The model under review builds one solid part; all positions refer to its coordinate system, in mm. A direction names the side the tool comes from. Coordinates: 2 decimals unless noted, no trailing zeros. Write each loop counter-clockwise with the first axis right and the second up, starting at its lowest first coordinate (ties: lowest second). Pieces come first, ordered by that corner, then holes. Notation, with made-up numbers: (-9.75, 7) -> (9.25, 7) arc R21 ccw to (9.25, 36) -> close; hole circle Ø6 at (67, 69). An arc over 180 degrees is marked (long way). Write each question's results on one line, items separated by ' | '.
```python
from build123d import *

# Parameters (mm, degrees)
F0_W     = 80
F0_H     = 180
F1_DEPTH = 15
F2_W     = 50
F2_H     = 2
F3_DEPTH = 180
F4_ANGLE = 90
F5_ANGLE = 90
F6_DEPTH = 25
F9_DEPTH = 80.001


with BuildPart() as f1:
    # F0 (on Top) → F1 (new body)
    with BuildSketch(Plane.XY):
        Rectangle(F0_W, F0_H)
    extrude(amount=F1_DEPTH)

    # F2 (on face) → F3 (intersect, through all)
    with BuildSketch(Plane.XZ.offset(90)):
        with BuildLine():
            Line((-38, 15), (-40, 15))
            ThreePointArc((-40, 15), (-35.6066017178, 4.3933982822), (-25, 0))
            Line((-25, 0), (-25, 2))
            ThreePointArc((-25, 2), (-34.1923881554, 5.8076118446), (-38, 15))
        make_face()
        with Locations((0, 1)):
            Rectangle(F2_W, F2_H)
        with BuildLine():
            Line((25, 2), (25, 0))
            ThreePointArc((25, 0), (35.6066017178, 4.3933982822), (40, 15))
            Line((40, 15), (38, 15))
            ThreePointArc((38, 15), (34.1923881554, 5.8076118446), (25, 2))
        make_face()
    extrude(amount=-F3_DEPTH, mode=Mode.INTERSECT)

    # F2 (on face) → F4 (revolve)
    with BuildSketch(Plane.XZ.offset(90)):
        with BuildLine():
            Line((25, 2), (25, 0))
            ThreePointArc((25, 0), (35.6066017178, 4.3933982822), (40, 15))
            Line((40, 15), (38, 15))
            ThreePointArc((38, 15), (34.1923881554, 5.8076118446), (25, 2))
        make_face()
    revolve(axis=Axis((12.5, -90, 8.5), (0, 0, -1)), revolution_arc=F4_ANGLE)

    # F2 (on face) → F5 (revolve)
    with BuildSketch(Plane.XZ.offset(90)):
        with BuildLine():
            Line((-38, 15), (-40, 15))
            ThreePointArc((-40, 15), (-35.6066017178, 4.3933982822), (-25, 0))
            Line((-25, 0), (-25, 2))
            ThreePointArc((-25, 2), (-34.1923881554, 5.8076118446), (-38, 15))
        make_face()
    revolve(axis=Axis((-12.5, -90, 8.5), (0, 0, 1)), revolution_arc=F5_ANGLE)

    # F6 (add, through all): a face of the model
    f6_faces = [f1.faces().sort_by_distance(p)[0] for p in [
        (-12.5, -111.8423881554, 5.6576118446),
    ]]
    extrude(f6_faces, amount=F6_DEPTH)

    # F8 (on face) → F9 (cut, through all)
    with BuildSketch(Plane.YZ.offset(40)):
        with BuildLine():
            Line((90, 7.6), (90, 15))
            Line((90, 15), (36, 15))
            ThreePointArc((36, 15), (55.6606293116, 9.4655638465), (76, 7.6))
            Line((76, 7.6), (90, 7.6))
        make_face()
    extrude(amount=-F9_DEPTH, mode=Mode.SUBTRACT)


solid = f1.part
```
Q1. For line 1 (Z direction, x = -7, y = 31); line 2 (X direction, y = 78, z = 4); line 3 (X direction, y = 76.5, z = 6.5), list the stretches that pass through material, from the lowest coordinate up. Write a range as from..to.
Solution:
line 1: 0..2 | line 2: -35.2..-31.93, 31.93..35.2 | line 3: -37.36..-34.84, 34.84..37.36
Q2. Machinability: for faces 1 (the flat face through (0, -1, 0)), 2 (the cylindrical face through (21.435, -98.741, 0.986)), 3 (the cylindrical face through (-34.091, -1.26, 5.707)), which of the approach directions +Z, -Z, +X, -X, +Y, -Y give a long, thin tool a straight path to every point of the face, cutting with its end or side? Answer none if there is none.
Solution:
face 1: -Z, +X, -X, +Y, -Y | face 2: +Z, -Z | face 3: +Z, +Y
Q3. Clearance check with flat-ended pins moving along their axes: P1, Ø0.6, axis at x = 5.5, z = 1, coming from the -Y side; P2, Ø0.7, axis at x = -37, y = 85.5, coming from the +Z side; P3, Ø1.5, axis at y = -27.5, z = 10.5, coming from the -X side; P4, Ø4, axis at x = -26.5, y = 8.5, coming from the -Z side. State where each tip first meets the part, or that it passes through.
Solution:
P1: y = -108.61 | P2: z = 7.6 | P3: x = -39.52 | P4: z = 0
Q4. Add section B-B (y = -61.5). Write out the cut boundary in (x, z), plus the area to 3 significant figures.
Solution:
outline: (-40, 15) arc R15 ccw to (-25, 0) -> (25, 0) arc R15 ccw to (40, 15) -> (38, 15) arc R13 cw to (25, 2) -> (-25, 2) arc R13 cw to (-38, 15) -> close | area: 188 mm²
Q5. Draft analysis for pull direction X (two halves, no side actions). For faces 4 (the cylindrical face through (-0.175, -111.591, 5.707)), 5 (the cylindrical face through (35.49, -1.26, 4.28)), 6 (the flat face through (-0.2, 90, 1.8)), 7 (the cylindrical face through (-21.435, -98.741, 1.014)), state which applies: pulls with the +X half, pulls with the -X half, needs draft (parallel to the pull), parting line crosses it, or undercut.
Solution:
face 4: undercut | face 5: pulls with the +X half | face 6: needs draft | face 7: undercut
Q6. Add section A-A (x = 4). Write out the cut boundary in (y, z), plus the area to 3 significant figures.
Solution:
outline: (-117.5, 15) arc R15 ccw to (-102.5, 0) -> (-102.5, 2) arc R13 cw to (-115.5, 15) -> close; (-90, 0) -> (90, 0) -> (90, 2) -> (-90, 2) -> close | area: 404 mm²
